Can you work these out from the model? Positions are in its coordinate system, mm. Face numbers are marked on the shaded views. A direction names the side the tool comes from. Round coordinates to 2 decimals unless told otherwise and drop trailing zeros. Write each loop counter-clockwise with the first axis right and the second up, starting at its lowest first coordinate (ties: lowest second). Pieces come first, ordered by that corner, then holes. Notation, with made-up numbers: M 37,3.5 L 60,3.5 A24 ccw 60,42.5 Z; hole C 6.25,-33.75 d4. An arc over 180 degrees is marked long. Answer in a Markdown table with one row per item. Add a question column.
(1) Suppose I cut it at D-D, the plane y = -3. Write out the boundary of the cut face in (x, z), then the cut area to 3 significant figures.
(2) Suppose I cut it at C-C, the plane y = 2.75. Write out the boundary of the cut face in (x, z).
(3) Suppose I cut it at B-B, the plane y = -0.5. Write out the boundary of the cut face in (x, z).
(4) If I drill on probe 1 along X at (y, z) = (-1, 1.9); probe 2 along X at (y, z) = (1.5, 0.6); probe 3 along Y at (x, z) = (18.5, 3.3), over which ranges is the centre line in solid material (lowest first)?
(5) For the marked faces 1 and 2, which set-ups out of +Z, -Z, +X, -X, +Y, -Y let a thin tool reach every point of the face, with its end or its side?
(6) Suppose I cut it at A-A, the plane z = 3.2. Write out the boundary of the cut face in (x, y).
(7) If we mould it in two halves opening along Y, with no side actions, what happens to the marked faces 3, 4, 5 and 6? For each: released by +Y, released by -Y, zero draft, split by the parting line, or undercut.
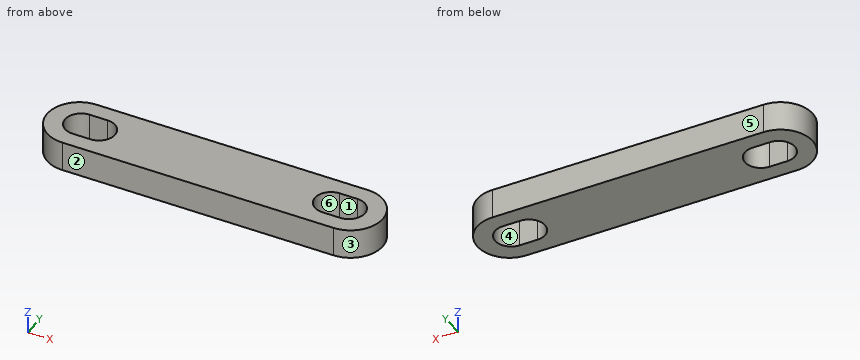
from build123d import *

# Parameters (mm, degrees)
SALIENTE_EXTRUIR2_DEPTH = 4.2


with BuildPart() as part:
    # Croquis1 → Saliente-Extruir2 (new body)
    with BuildSketch(Plane.XY):
        with BuildLine():
            Line((19, 4.5), (-19, 4.5))
            ThreePointArc((-19, 4.5), (-23.5, 0), (-19, -4.5))
            Line((-19, -4.5), (19, -4.5))
            ThreePointArc((19, -4.5), (23.5, 0), (19, 4.5))
        make_face()
        with BuildLine():
            Line((18.75, 2.25), (16.25, 2.25))
            ThreePointArc((16.25, 2.25), (14, 0), (16.25, -2.25))
            Line((16.25, -2.25), (18.75, -2.25))
            ThreePointArc((18.75, -2.25), (21, 0), (18.75, 2.25))
        make_face(mode=Mode.SUBTRACT)
        with BuildLine():
            Line((-16.25, 2.25), (-18.75, 2.25))
            ThreePointArc((-18.75, 2.25), (-21, 0), (-18.75, -2.25))
            Line((-18.75, -2.25), (-16.25, -2.25))
            ThreePointArc((-16.25, -2.25), (-14, 0), (-16.25, 2.25))
        make_face(mode=Mode.SUBTRACT)
    extrude(amount=SALIENTE_EXTRUIR2_DEPTH)


solid = part.part
Calculated:
| question | item | result |
|---|---|---|
| 1 | outline | M -22.35,0 L 22.35,0 L 22.35,4.2 L -22.35,4.2 Z |
| 1 | area | 188 mm² |
| 2 | outline | M -22.56,0 L 22.56,0 L 22.56,4.2 L -22.56,4.2 Z |
| 3 | outline | M -23.47,0 L -20.94,0 L -20.94,4.2 L -23.47,4.2 Z; M -14.06,0 L 14.06,0 L 14.06,4.2 L -14.06,4.2 Z; M 20.94,0 L 23.47,0 L 23.47,4.2 L 20.94,4.2 Z |
| 4 | probe 1 | -23.39 to -20.77, -14.23 to 14.23, 20.77 to 23.39 |
| 4 | probe 2 | -23.24 to -20.43, -14.57 to 14.57, 20.43 to 23.24 |
| 4 | probe 3 | -4.5 to -2.25, 2.25 to 4.5 |
| 5 | face 1 | +Z, -Z |
| 5 | face 2 | +Z, -Z, +X, -X, -Y |
| 6 | outline | M -19,-4.5 L 19,-4.5 A4.5 ccw 19,4.5 L -19,4.5 A4.5 ccw Z; hole M -18.75,-2.25 L -16.25,-2.25 A2.25 ccw -16.25,2.25 L -18.75,2.25 A2.25 ccw Z; hole M 16.25,-2.25 L 18.75,-2.25 A2.25 ccw 18.75,2.25 L 16.25,2.25 A2.25 ccw Z |
| 7 | face 3 | split by the parting line |
| 7 | face 4 | undercut |
| 7 | face 5 | released by +Y |
| 7 | face 6 | undercut |
